Could you check a few things on this model? Use its own coordinates, in mm. A direction names the side the tool comes from. Give positions to 0.01 mm unless a question says otherwise; leave off trailing zeros. Write each loop counter-clockwise with the first axis right and the second up, starting at its lowest first coordinate (ties: lowest second). Pieces come first, ordered by that corner, then holes. Notation, with made-up numbers: (-36, 34.5) -> (-7, 34.5) arc R35 cw to (-7, 68.5) -> close; hole circle Ø9 at (43.25, 63.5). An arc over 180 degrees is marked (long way). Write item = value, one per line. Start each with the question number.
Autodesk Inventor part; units mm, degrees
ref_plane "YZ Plane" through (0, 0, 0) normal (1, 0, 0) x (0, 1, 0)
ref_plane "XZ Plane" through (0, 0, 0) normal (0, 1, 0) x (-1, 0, 0)
ref_plane "XY Plane" through (0, 0, 0) normal (0, 0, 1) x (1, 0, 0)
sketch "Sketch1" plane through (0, 0, 0) normal (0, 1, 0) x (-1, 0, 0)
  line L0 (0, 0) -> (19.05, 0)
  line L1 (0, 0) -> (-19.05, 0)
  line L2 (0, 0) -> (0, -19.05)
  circle A0 centre (-19.05, 0) radius 1.5
  circle A1 centre (19.05, 0) radius 1.5
  circle A2 centre (0, -19.05) radius 1.5
  line L3 (0, -20.55) -> (0, -22.55)
  line L4 (0, -22.55) -> (5, -22.55)
  line L5 (5, -22.55) -> (5, -27.55)
  line L6 (5, -27.55) -> (-5, -27.55)
  line L7 (-5, -27.55) -> (-5, -22.55)
  line L8 (-5, -22.55) -> (0, -22.55)
  circle A3 centre (0, 0) radius 30
  dimension "d6" = 3
  dimension "d0" = 19.05
  dimension "d1" = 19.05
  dimension "d2" = 19.05
  dimension "d4" = 3
  dimension "d5" = 3
  dimension "d7" = 2
  dimension "d8" = 5
  dimension "d9" = 5
  dimension "d10" = 10
  dimension "d11" = 60
extrude "Extrusion1" add sketch "Sketch1" along normal blind 1.5 contours L4 L5 L6 L7 L8 | A3
sketch "Sketch2" plane through (0, 1.5, 0) normal (0, 1, 0) x (1, 0, 0)
  line L0 (0, 0) -> (0, 22)
  line L1 (0, 22) -> (-5, 22)
  line L2 (-5, 22) -> (-5, 27)
  line L3 (-5, 27) -> (0, 27)
  line L4 (0, 27) -> (5, 27)
  line L5 (5, 27) -> (5, 22)
  line L6 (5, 22) -> (0, 22)
  line L7 (-11, 19.0526) -> (-15.3301, 16.5526)
  line L8 (-15.3301, 16.5526) -> (-17.8301, 20.8827)
  line L9 (-17.8301, 20.8827) -> (-13.5, 23.3827)
  line L10 (-13.5, 23.3827) -> (-9.1699, 25.8827)
  line L11 (-9.1699, 25.8827) -> (-6.6699, 21.5526)
  line L12 (-6.6699, 21.5526) -> (-11, 19.0526)
  line L13 (-19.0526, 11) -> (-21.5526, 6.6699)
  line L14 (-21.5526, 6.6699) -> (-25.8827, 9.1699)
  line L15 (-25.8827, 9.1699) -> (-23.3827, 13.5)
  line L16 (-23.3827, 13.5) -> (-20.8827, 17.8301)
  line L17 (-20.8827, 17.8301) -> (-16.5526, 15.3301)
  line L18 (-16.5526, 15.3301) -> (-19.0526, 11)
  line L19 (-22, 0) -> (-22, -5)
  line L20 (-22, -5) -> (-27, -5)
  line L21 (-27, -5) -> (-27, 0)
  line L22 (-27, 0) -> (-27, 5)
  line L23 (-27, 5) -> (-22, 5)
  line L24 (-22, 5) -> (-22, 0)
  line L25 (-19.0526, -11) -> (-16.5526, -15.3301)
  line L26 (-16.5526, -15.3301) -> (-20.8827, -17.8301)
  line L27 (-20.8827, -17.8301) -> (-23.3827, -13.5)
  line L28 (-23.3827, -13.5) -> (-25.8827, -9.1699)
  line L29 (-25.8827, -9.1699) -> (-21.5526, -6.6699)
  line L30 (-21.5526, -6.6699) -> (-19.0526, -11)
  line L31 (-11, -19.0526) -> (-6.6699, -21.5526)
  line L32 (-6.6699, -21.5526) -> (-9.1699, -25.8827)
  line L33 (-9.1699, -25.8827) -> (-13.5, -23.3827)
  line L34 (-13.5, -23.3827) -> (-17.8301, -20.8827)
  line L35 (-17.8301, -20.8827) -> (-15.3301, -16.5526)
  line L36 (-15.3301, -16.5526) -> (-11, -19.0526)
  line L37 (0, -22) -> (5, -22)
  line L38 (5, -22) -> (5, -27)
  line L39 (5, -27) -> (0, -27)
  line L40 (0, -27) -> (-5, -27)
  line L41 (-5, -27) -> (-5, -22)
  line L42 (-5, -22) -> (0, -22)
  line L43 (11, -19.0526) -> (15.3301, -16.5526)
  line L44 (15.3301, -16.5526) -> (17.8301, -20.8827)
  line L45 (17.8301, -20.8827) -> (13.5, -23.3827)
  line L46 (13.5, -23.3827) -> (9.1699, -25.8827)
  line L47 (9.1699, -25.8827) -> (6.6699, -21.5526)
  line L48 (6.6699, -21.5526) -> (11, -19.0526)
  line L49 (19.0526, -11) -> (21.5526, -6.6699)
  line L50 (21.5526, -6.6699) -> (25.8827, -9.1699)
  line L51 (25.8827, -9.1699) -> (23.3827, -13.5)
  line L52 (23.3827, -13.5) -> (20.8827, -17.8301)
  line L53 (20.8827, -17.8301) -> (16.5526, -15.3301)
  line L54 (16.5526, -15.3301) -> (19.0526, -11)
  line L55 (22, 0) -> (22, 5)
  line L56 (22, 5) -> (27, 5)
  line L57 (27, 5) -> (27, 0)
  line L58 (27, 0) -> (27, -5)
  line L59 (27, -5) -> (22, -5)
  line L60 (22, -5) -> (22, 0)
  line L61 (19.0526, 11) -> (16.5526, 15.3301)
  line L62 (16.5526, 15.3301) -> (20.8827, 17.8301)
  line L63 (20.8827, 17.8301) -> (23.3827, 13.5)
  line L64 (23.3827, 13.5) -> (25.8827, 9.1699)
  line L65 (25.8827, 9.1699) -> (21.5526, 6.6699)
  line L66 (21.5526, 6.6699) -> (19.0526, 11)
  line L67 (11, 19.0526) -> (6.6699, 21.5526)
  line L68 (6.6699, 21.5526) -> (9.1699, 25.8827)
  line L69 (9.1699, 25.8827) -> (13.5, 23.3827)
  line L70 (13.5, 23.3827) -> (17.8301, 20.8827)
  line L71 (17.8301, 20.8827) -> (15.3301, 16.5526)
  line L72 (15.3301, 16.5526) -> (11, 19.0526)
  dimension "d14" = 22
  dimension "d15" = 5
  dimension "d16" = 5
  dimension "d17" = 5
  dimension "d18" = 5
  dimension "d21" = 360
extrude "Extrusion2" add sketch "Sketch2" along normal blind 2.5
properties part number "TSSP Receiver"
(1) Imagine slicing it at A-A (z = 0). Please give me the cut outline in (x, y).
(2) We'd pull the mould along X, two halves only. Please class faces 1 (the flat face through (0, 3, 22)), 2 (the flat face through (-24, 3, 5)), 3 (the flat face through (-23.687, 2.732, -7.902)): released by +X, released by -X, zero draft, split by the parting line, or undercut.
(3) Imagine slicing it at B-B (y = 2.4). State how many separate pieces and enclosed holes the cut face has, then the cut area to 3 significant figures.
(4) I'm going to push flat-ended pins straight in: pin 1 (2 mm diameter, centred on x = -0.5, y = 3, fed in from +Z); pin 2 (1.2 mm diameter, centred on y = 2.5, z = 0.5, fed in from -X); pin 3 (1 mm diameter, centred on x = -20.5, y = 1.5, fed in from -Z). Where does each tip first touch, or does it pass through?
(5) Imagine slicing it at D-D (x = 4). Please give me the cut outline in (y, z), then the cut area to 3 significant figures.
(6) If I drill on line 1 along Z through (x, y) = (2.5, 2.8); line 2 along Z through (x, y) = (0, 0.7); line 3 along Y through (x, z) = (6.5, 5.5), over which ranges is the centre line in solid material (lowest first)? Write a range as from..to.
(7) Imagine slicing it at C-C (x = -19.05). Please give me the cut outline in (y, z), then the cut area to 3 significant figures.
(8) On a 3-axis mill with a long thin cutter (end or side, diameter ignored), from which of +Z, -Z, +X, -X, +Y, -Y can I reach the whole of each face in a straight line? I mean faces 4 (the flat face through (-16.563, 2.732, -18.687)), 5 (the flat face through (-7.94, 2.73, -23.75)), 6 (the flat face through (-7.902, 2.732, 23.687)). Say none if no direction works.
Answers below:
q1.outline = (-30, 0) -> (-20.55, 0) -> (-20.55, 1.5) -> (-22, 1.5) -> (-22, 4) -> (-27, 4) -> (-27, 1.5) -> (-30, 1.5) -> close; (-17.55, 0) -> (17.55, 0) -> (17.55, 1.5) -> (-17.55, 1.5) -> close; (20.55, 0) -> (30, 0) -> (30, 1.5) -> (27, 1.5) -> (27, 4) -> (22, 4) -> (22, 1.5) -> (20.55, 1.5) -> close
q2.face_1 = undercut
q2.face_2 = zero draft
q2.face_3 = released by -X
q3.separate_pieces = 12
q3.enclosed_holes = 0
q3.area = 600 mm^2
q4.pin_1 = 27
q4.pin_2 = -27
q4.pin_3 = -22.36
q5.outline = (0, -29.73) -> (1.5, -29.73) -> (1.5, -27) -> (4, -27) -> (4, -22) -> (1.5, -22) -> (1.5, 22) -> (4, 22) -> (4, 27) -> (1.5, 27) -> (1.5, 29.73) -> (0, 29.73) -> close
q5.area = 114 mm^2
q6.line_1 = -27..-22, 22..27
q6.line_2 = -30..-20.55, -17.55..30
q6.line_3 = 0..1.5
q7.outline = (0, -23.18) -> (1.5, -23.18) -> (1.5, -16.77) -> (4, -16.77) -> (4, -11) -> (1.5, -11) -> (1.5, -1.5) -> (0, -1.5) -> close; (0, 1.5) -> (1.5, 1.5) -> (1.5, 11) -> (4, 11) -> (4, 16.77) -> (1.5, 16.77) -> (1.5, 23.18) -> (0, 23.18) -> close
q7.area = 93.9 mm^2
q8.face_4 = +Y
q8.face_5 = -Z, +Y
q8.face_6 = +Z, +Y
